Here's how the part is built. I have some questions about the finished solid (model axes, mm). Coordinates: 2 decimals unless noted, no trailing zeros. Write each loop counter-clockwise with the first axis right and the second up, starting at its lowest first coordinate (ties: lowest second). Pieces come first, ordered by that corner, then holes.
Item 1: If we section it at B-B (y = 150.5): Please give me the cut outline in (x, z), then the cut area to 3 significant figures.
Item 2: If we section it at C-C (x = -66.5): Please give me the cut outline in (y, z).
Item 3: I'm going to push flat-ended pins straight in: pin 1 Ø2.5 at (x, z) = (-74, 6.5) entering from +Y; pin 2 Ø2.5 at (y, z) = (47, 7.5) entering from -X; pin 3 Ø1.5 at (y, z) = (147, 8.5) entering from +X. Where does each tip first touch, or does it pass through?
Item 4: If I drill on line 1 (Y direction, x = -72.5, z = 8); line 2 (X direction, y = 41.5, z = 6.4), over which ranges is the centre line in solid material (lowest first)?
Item 5: If we section it at A-A (z = 8.65): Please give me the cut outline in (x, y).
Autodesk Inventor part; units mm, degrees
ref_plane "YZ Plane" through (0, 0, 0) normal (1, 0, 0) x (0, 1, 0)
ref_plane "XZ Plane" through (0, 0, 0) normal (0, 1, 0) x (-1, 0, 0)
ref_plane "XY Plane" through (0, 0, 0) normal (0, 0, 1) x (1, 0, 0)
sketch "Skizze3" plane through (0, 0, 0) normal (0, 0, 1) x (1, 0, 0)
  line L0 (0, 0) -> (0, 200)
  line L1 (0, 200) -> (-20, 200)
  line L2 (-20, 200) -> (-20, 220)
  line L3 (-20, 220) -> (-120, 220)
  line L4 (-120, 220) -> (-120, 200)
  line L5 (-120, 200) -> (-140, 200)
  line L6 (-140, 200) -> (-140, 160)
  line L7 (-140, 160) -> (-120, 160)
  line L8 (-120, 160) -> (-120, 140)
  line L9 (-120, 140) -> (-140, 140)
  line L10 (-140, 140) -> (-140, 160)
  line L11 (-140, 160) -> (-360, 160)
  line L12 (-360, 160) -> (-360, 140)
  line L13 (-360, 140) -> (-380, 140)
  line L14 (-380, 140) -> (-380, 60)
  line L15 (-380, 60) -> (-360, 60)
  line L16 (-360, 60) -> (-360, 40)
  line L17 (-360, 40) -> (-140, 40)
  line L18 (-140, 40) -> (-140, 60)
  line L19 (-140, 60) -> (-120, 60)
  line L20 (-120, 60) -> (-120, 40)
  line L21 (-120, 40) -> (-140, 40)
  line L22 (-140, 40) -> (-140, 0)
  line L23 (-140, 0) -> (-120, 0)
  line L24 (-120, 0) -> (-120, -20)
  line L25 (-120, -20) -> (-20, -20)
  line L26 (-20, -20) -> (-20, 0)
  line L27 (-20, 0) -> (0, 0)
  dimension "d4" = 200
  dimension "d5" = 20
  dimension "d6" = 20
  dimension "d7" = 100
  dimension "d8" = 20
  dimension "d9" = 20
  dimension "d10" = 20
  dimension "d11" = 40
  dimension "d12" = 220
  dimension "d13" = 20
  dimension "d14" = 20
  dimension "d15" = 220
  dimension "d16" = 80
  dimension "d17" = 20
  dimension "d18" = 20
  dimension "d19" = 20
  dimension "d20" = 100
  dimension "d21" = 20
  dimension "d22" = 20
  dimension "d23" = 40
ref_plane "Arbeitsebene1" through (0, 0, 5) normal (0, 0, 1) x (1, 0, 0)
sketch "Skizze4" plane through (0, 0, 5) normal (0, 0, 1) x (1, 0, 0)
  line L0 (-20, 0) -> (-20, 200)
  line L1 (-20, 200) -> (-120, 200)
  line L2 (-120, 200) -> (-120, 0)
  line L3 (-120, 0) -> (-20, 0)
  line L4 (-59.5, 0) -> (-59.5, 3.5)
  line L5 (-59.5, 3.5) -> (-80.5, 3.5)
  line L6 (-80.5, 3.5) -> (-80.5, 0)
  line L7 (-20, 39.5) -> (-23.5, 39.5)
  line L8 (-23.5, 39.5) -> (-23.5, 60.5)
  line L9 (-23.5, 60.5) -> (-20, 60.5)
  point P0 (0, 0)
  point P1 (-23.5, 50)
  dimension "d26" = 3.5
  dimension "d27" = 39.5
  dimension "d28" = 21
  dimension "d29" = 39.5
  dimension "d36" = 3.5
  dimension "d37" = 21
  dimension "d38" = 39.5
extrude "Extrusion5" add sketch "Skizze4" along normal blind 5
ref_plane "Arbeitsebene2" through (-70, 0, 10) normal (1, 0, 0) x (0, 1, 0)
ref_plane "Arbeitsebene3" through (-120, 100, 10) normal (0, -1, 0) x (1, 0, 0)
extrude "Extrusion6" cut sketch "Skizze4" along normal blind 5 contours L7 L8 L9 L0 | L3 L6 L5 L4
mirror "Spiegeln1" about plane through (-70, 0, 10) normal (1, 0, 0) of "Extrusion6"
mirror "Spiegeln2" about plane through (-120, 100, 10) normal (0, -1, 0) of "Extrusion6", "Spiegeln1"
equation "\"d37\" = d28"
equation "\"d38\" = d27"
properties part number "BT003_trajan20_21"
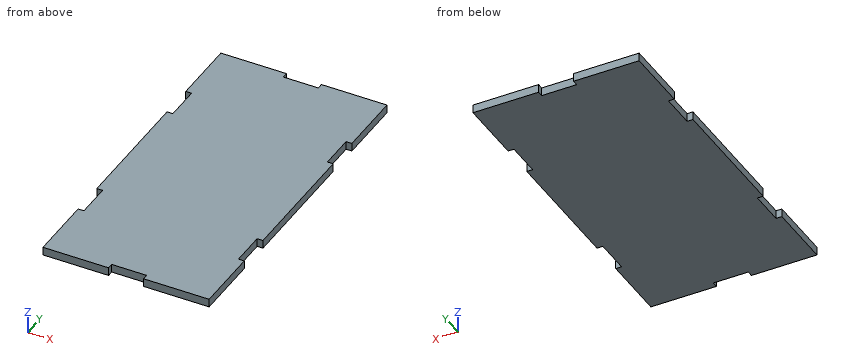
Answer list:
1. outline: (-116.5, 5) - (-23.5, 5) - (-23.5, 10) - (-116.5, 10) - close
1. area: 465 mm2
2. outline: (3.5, 5) - (196.5, 5) - (196.5, 10) - (3.5, 10) - close
3. pin 1: stops at y = 196.5
3. pin 2: stops at x = -116.5
3. pin 3: stops at x = -23.5
4. line 1: y = 3.5 to 196.5
4. line 2: x = -116.5 to -23.5
5. outline: (-120, 0) - (-80.5, 0) - (-80.5, 3.5) - (-59.5, 3.5) - (-59.5, 0) - (-20, 0) - (-20, 39.5) - (-23.5, 39.5) - (-23.5, 60.5) - (-20, 60.5) - (-20, 139.5) - (-23.5, 139.5) - (-23.5, 160.5) - (-20, 160.5) - (-20, 200) - (-59.5, 200) - (-59.5, 196.5) - (-80.5, 196.5) - (-80.5, 200) - (-120, 200) - (-120, 160.5) - (-116.5, 160.5) - (-116.5, 139.5) - (-120, 139.5) - (-120, 60.5) - (-116.5, 60.5) - (-116.5, 39.5) - (-120, 39.5) - close
